Source: CAD feature listing. Evaluate the final solid. Frame: model axes, mm. A direction names the side the tool comes from. Coordinates: 2 decimals unless noted, no trailing zeros. Write each loop counter-clockwise with the first axis right and the second up, starting at its lowest first coordinate (ties: lowest second). Pieces come first, ordered by that corner, then holes. Notation, with made-up numbers: (86, -30) -> (110, -30) arc R17 cw to (110, -25) -> close; hole circle Ø11 at (-16, 7.5). An arc over 180 degrees is marked (long way). One line per item, written item: value. Start each with the question number.
1. Section query A-A, the plane x = -9. Output: boundary loops of the cut face in (y, z), and give its area (3 significant figures).
2. Line query: line 1 (X direction, y = -13.25, z = 0) (1 decimal); line 2 (X direction, y = -129.5, z = 6.5) (3 decimals); line 3 (Y direction, x = 33.5, z = -3). Output: solid intervals per line, ascending.
3. Section query B-B, the plane y = -131.5. State how many separate pieces and enclosed holes the cut face has, and give its area (3 significant figures).
4. Access query for faces 4 (the cylindrical face through (-25, -12.88, 0.19)), 5 (the flat face through (-1, -153.365, 10)), 6 (the conical face through (31.59, -123.34, 9.93)). Directions: +Z, -Z, +X, -X, +Y, -Y. A direction counts if a zero-diameter tool reaches every point of the face in a straight line with its end or side. Return the directions, or none.
5. First-contact query: P1, Ø5, axis at x = 22.5, z = -3.5, coming from the -Y side; P2, Ø7, axis at x = 20.64, z = 0, coming from the +Y side. Flat tips, straight axial feed; report the tip coordinate or a pass-through.
6. Mould query, pull axis Y, two halves, no side actions, for faces 1 (the conical face through (-31.91, -123.34, 9.93)), 2 (the conical face through (19.914, -27.567, 0.228)), 3 (the cylindrical face through (16.277, -12.878, 0.192)). Classes: released by +Y, released by -Y, zero draft, split by the parting line, or undercut.
from build123d import *

# Parameters (mm, degrees)
F0_W           = 82.55
F0_H           = 38.1
F1_DEPTH       = 153.3652
F2_SIZE2       = 20.0152
F2_SIZE        = 20.0152
F5_D           = 8.72998
F5_DEPTH       = 25.4
F5_TIP         = 2.6227505934
F5_ON_F4_D     = 8.72998
F5_ON_F4_DEPTH = 25.4
F5_ON_F4_TIP   = 2.6227505934


with BuildPart() as f1:
    # F0 (on Front) → F1 (new body)
    with BuildSketch(Plane.XZ):
        Rectangle(F0_W, F0_H)
    extrude(amount=F1_DEPTH)

    # F2
    f2_edges = [f1.edges().sort_by_distance(p)[0] for p in [
        (0, -153.3652, -19.05),
    ]]
    chamfer(f2_edges, length=F2_SIZE, length2=F2_SIZE2)

    # F5
    with Locations(Plane(origin=(0, -76.2, -76.2), x_dir=(1, 0, 0), z_dir=(0, -0.7071067812, -0.7071067812))):
        with Locations((-31.75, 94.9751887364), (31.75, 94.9751887364)):
            Hole(F5_D / 2, depth=F5_DEPTH)
            with Locations((0, 0, -(F5_DEPTH + F5_TIP / 2))):  # 118° drill point
                Cone(0, F5_D / 2, F5_TIP, mode=Mode.SUBTRACT)

    # F5 on F4
    with Locations(Plane(origin=(0, 0, 0), x_dir=(-1, 0, 0), z_dir=(0, 1, 0))):
        with Locations((-20.6375, 0), (20.6375, 0)):
            Hole(F5_ON_F4_D / 2, depth=F5_ON_F4_DEPTH)
            with Locations((0, 0, -(F5_ON_F4_DEPTH + F5_ON_F4_TIP / 2))):  # 118° drill point
                Cone(0, F5_ON_F4_D / 2, F5_ON_F4_TIP, mode=Mode.SUBTRACT)


solid = f1.part
Computed values:
1. outline: (-153.37, 0.97) -> (-133.35, -19.05) -> (0, -19.05) -> (0, 19.05) -> (-153.37, 19.05) -> close
1. area: 5,640 mm²
2. line 1: x = -41.3 to -25, -16.3 to 16.3, 25 to 41.3
2. line 2: x = -41.275 to -35.949, -27.551 to 27.551, 35.949 to 41.275
2. line 3: y = -149.4 to -142.97, -131.66 to 0
3. separate pieces: 1
3. enclosed holes: 2
3. area: 2,980 mm²
4. face 4: +Y
4. face 5: +Z, -Z, +X, -X, -Y
4. face 6: none
5. P1: stops at y = -151.4
5. P2: stops at y = -25.92
6. face 1: undercut
6. face 2: released by +Y
6. face 3: zero draft
